The listing builds one solid part. Answer for the finished solid, in the listing's coordinates (mm). Round coordinates to 2 decimals unless told otherwise and drop trailing zeros. Order: outer loops, then holes, each group sorted by start corner. A loop starts at its lowest first (then second) coordinate and runs counter-clockwise, first axis right, second up. Notation, with made-up numbers: (66, -35) -> (115, -35) arc R8 cw to (115, -26) -> close; hole circle Ø11 at (-24, 35.5). An arc over 180 degrees is marked (long way). Return JSON: item names as keys, results as strings. Group by question number.
(1) The part is cut by section D-D (y = -3). Determine the outline of the cut face in (x, z), plus the area to 3 significant figures.
(2) The part is cut by section B-B (z = 0.35). Determine the outline of the cut face in (x, y).
(3) This flat-tipped pin is pushed along its axis until it touches: pin 1 (4 mm diameter, centred on x = -3, y = 9.5, fed in from +Z). Where does it stop, or does it pass through?
(4) The part is cut by section A-A (x = -1). Determine the outline of the cut face in (y, z), plus the area to 3 significant figures.
(5) Consider line 1 (Y direction, x = -0.75, z = 0.7); line 2 (Y direction, x = -3, z = 0.6); line 3 (X direction, y = -5.25, z = 0.15). Determine where each line is inside the solid, lowest interval first. Write a range as [from, to].
(6) The part is cut by section C-C (x = 3.5). Determine the outline of the cut face in (y, z).
from build123d import *

# Parameters (mm, degrees)
F0_W          = 11
F0_H          = 20
F1_DEPTH      = 1
F3_DEPTH      = 25.4
F3_DEPTH_BACK = 25.4


with BuildPart() as f1:
    # F0 (on Top) → F1 (new body)
    with BuildSketch(Plane.XY):
        with Locations((0, 3.033641)):
            Rectangle(F0_W, F0_H)
    extrude(amount=F1_DEPTH)

    # F2 (on face) → F3 (cut, two sides)
    with BuildSketch(Plane.XY.offset(1)) as f3_sk:
        with BuildLine():
            ThreePointArc((-5.5, -6.966359), (1.571068, -4.037426), (4.5, 3.033641))
            ThreePointArc((4.5, 3.033641), (1.571068, 10.104709), (-5.5, 13.033641))
            Line((-5.5, 13.033641), (-5.5, -6.966359))
        make_face()
    extrude(amount=-F3_DEPTH, mode=Mode.SUBTRACT)
    extrude(f3_sk.sketch, amount=-F3_DEPTH_BACK, mode=Mode.SUBTRACT)


solid = f1.part
Answer below:
{
 "1": {"outline": "(2.47, 0) -> (5.5, 0) -> (5.5, 1) -> (2.47, 1) -> close", "area": "3.03 mm²"},
 "2": {"outline": "(-5.5, -6.97) -> (5.5, -6.97) -> (5.5, 13.03) -> (-5.5, 13.03) arc R10 cw to (4.5, 3.03) arc R10 cw to start"},
 "3": {"pin 1": "passes through"},
 "4": {"outline": "(-6.97, 0) -> (-5.9, 0) -> (-5.9, 1) -> (-6.97, 1) -> close; (11.96, 0) -> (13.03, 0) -> (13.03, 1) -> (11.96, 1) -> close", "area": "2.14 mm²"},
 "5": {"line 1": "y = [-6.97, -5.77], [11.83, 13.03]", "line 2": "y = [-6.97, -6.65], [12.72, 13.03]", "line 3": "x = [0.1, 5.5]"},
 "6": {"outline": "(-6.97, 0) -> (-1.33, 0) -> (-1.33, 1) -> (-6.97, 1) -> close; (7.39, 0) -> (13.03, 0) -> (13.03, 1) -> (7.39, 1) -> close"}
}
